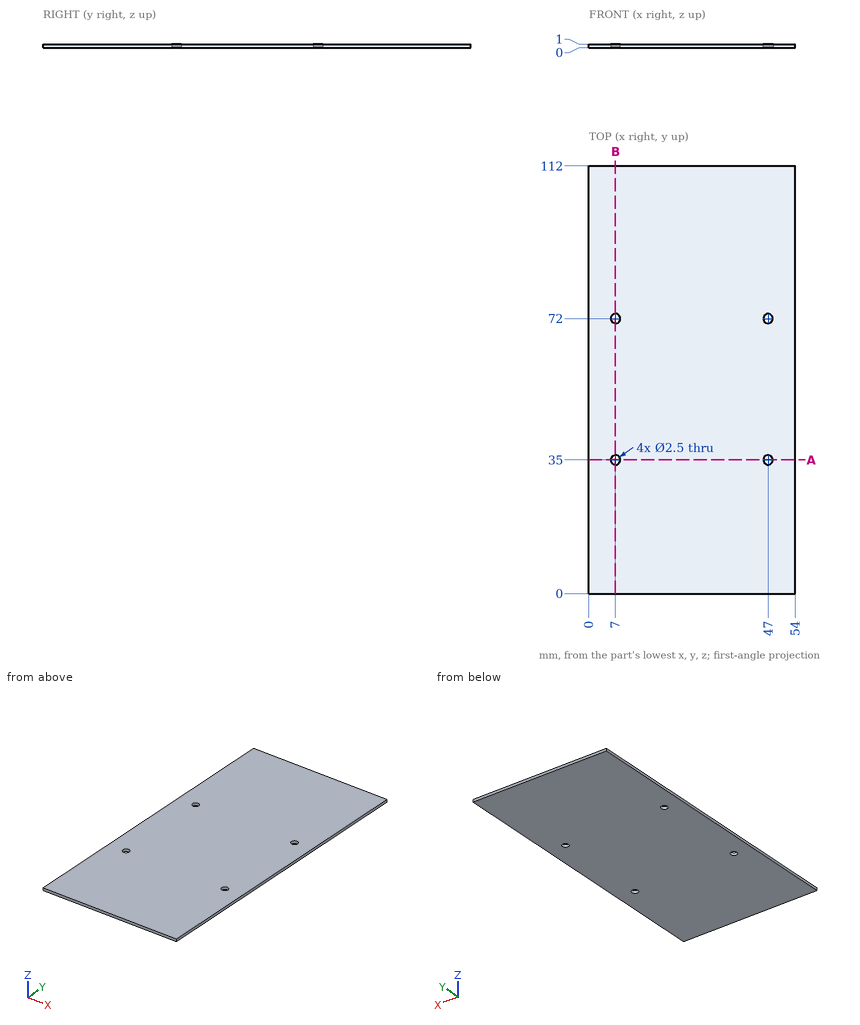
Check sheet for the drawn part. Datum: minimum x, y, z corner. Units: mm. Round coordinates to 2 decimals unless told otherwise and drop trailing zeros. Write each loop counter-clockwise with the first axis right and the second up, starting at its lowest first coordinate (ties: lowest second). Pieces come first, ordered by that corner, then holes. Notation, with made-up numbers: (31.25, 83.5) - (40.25, 83.5) arc R26 ccw to (40.25, 120.5) - close; hole circle Ø9 at (-3, 40.5). An arc over 180 degrees is marked (long way). Write each question's results on one line, items separated by ' | '.
(1) Sectioned sample at B-B, the plane x = 7. Enter the section's corners in (y, z).
Computed:
outline: (0, 0) - (33.75, 0) - (33.75, 1) - (0, 1) - close; (36.25, 0) - (70.75, 0) - (70.75, 1) - (36.25, 1) - close; (73.25, 0) - (112, 0) - (112, 1) - (73.25, 1) - close
(2) Sectioned sample at A-A, the plane y = 35. Enter the section's corners in (x, z).
Computed:
outline: (0, 0) - (5.75, 0) - (5.75, 1) - (0, 1) - close; (8.25, 0) - (45.75, 0) - (45.75, 1) - (8.25, 1) - close; (48.25, 0) - (54, 0) - (54, 1) - (48.25, 1) - close
(3) Depth check by flat-ended pin: pin 1 Ø1.5 at (x, y) = (47, 35) entering from -Z; pin 2 Ø12 at (x, y) = (38, 19) entering from -Z. Enter the tip coordinate at first touch or a pass-through.
Computed:
pin 1: passes through | pin 2: stops at z = 0
(4) Thickness scan on probe 1 along Y at (x, z) = (47, 0.6); probe 2 along X at (y, z) = (72, 0.35); probe 3 along Y at (x, z) = (8, 0.3). Record the ranges inside material, lowest first. Write a range as from..to.
Computed:
probe 1: y = 0..33.75, 36.25..70.75, 73.25..112 | probe 2: x = 0..5.75, 8.25..45.75, 48.25..54 | probe 3: y = 0..34.25, 35.75..71.25, 72.75..112
